Check sheet for the drawn part. Datum: minimum x, y, z corner. Units: mm. A direction names the side the tool comes from. Round coordinates to 2 decimals unless told otherwise and drop trailing zeros. Write each loop counter-clockwise with the first axis right and the second up, starting at its lowest first coordinate (ties: lowest second). Pieces come first, ordered by that corner, then holes. Notation, with made-up numbers: (6, 65) - (28, 65) arc R28 cw to (28, 95) - close; hole circle Ø10 at (-26, -33.75). An arc over 180 degrees is marked (long way). Answer as a JSON object with one key per item and string values.
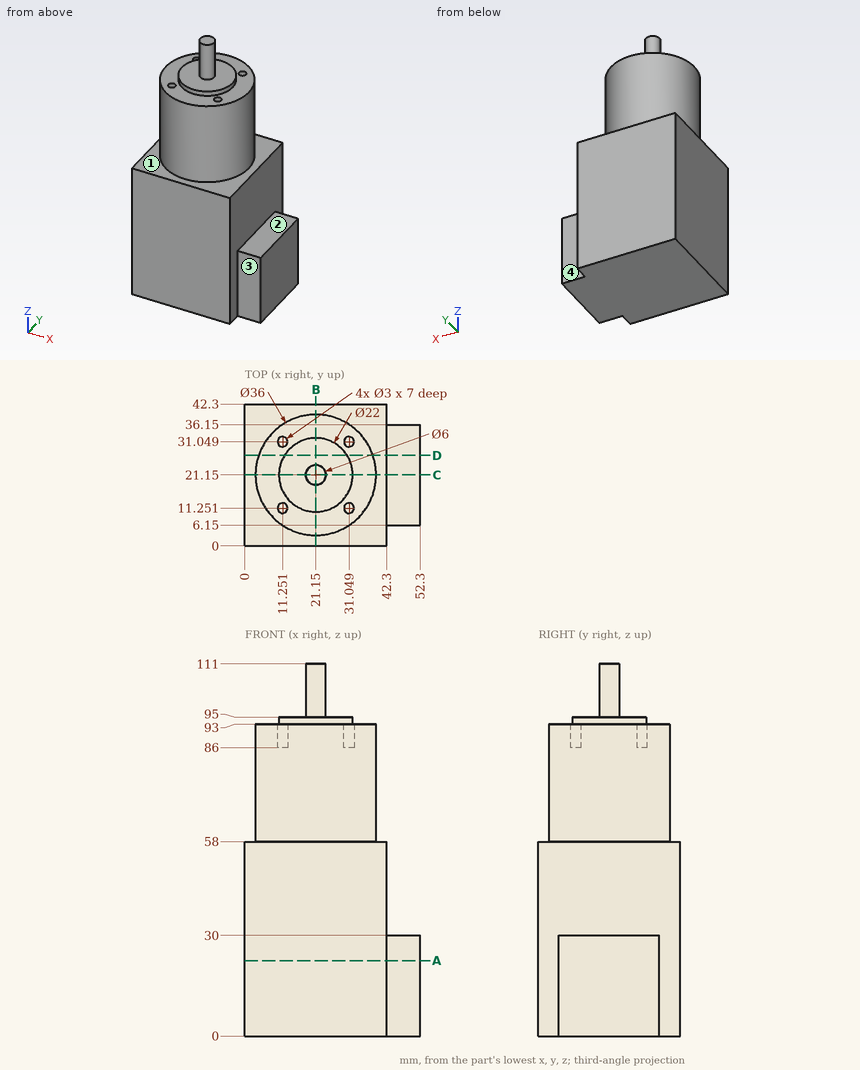
1. Cross-section at A-A (z = 22.5). Record the boundary of the cut face in (x, y), plus the area to 3 significant figures.
Completed:
{"outline": "(0, 0) - (42.3, 0) - (42.3, 6.15) - (52.3, 6.15) - (52.3, 36.15) - (42.3, 36.15) - (42.3, 42.3) - (0, 42.3) - close", "area": "2,090 mm^2"}
2. Material ranges on probe 1 along Z at (x, y) = (34, 6.5); probe 2 along Z at (x, y) = (26, 32); probe 3 along X at (y, z) = (5.5, 14.5), recorded low to high. Write a range as from..to.
Completed:
{"probe 1": "z = 0..58", "probe 2": "z = 0..93", "probe 3": "x = 0..42.3"}
3. Cross-section at B-B (x = 21.15). Record the boundary of the cut face in (y, z).
Completed:
{"outline": "(0, 0) - (42.3, 0) - (42.3, 58) - (39.15, 58) - (39.15, 93) - (32.15, 93) - (32.15, 95) - (24.15, 95) - (24.15, 111) - (18.15, 111) - (18.15, 95) - (10.15, 95) - (10.15, 93) - (3.15, 93) - (3.15, 58) - (0, 58) - close"}
4. Go/stop test with flat-tipped pins: pin 1 (5 mm diameter, centred on x = 48, z = 12.5, fed in from -Y); pin 2 (3.5 mm diameter, centred on x = 31.05, y = 11.25, fed in from +Z); pin 3 (1.5 mm diameter, centred on x = 31, y = 11.5, fed in from +Z). Record where each tip stops, or that it passes through.
Completed:
{"pin 1": "stops at y = 6.15", "pin 2": "stops at z = 93", "pin 3": "stops at z = 86"}
5. Access from +Z, -Z, +X, -X, +Y, -Y to the whole of each face (thin tool, end or side, straight path). Record for the marked faces 1, 2, 3 and 4.
Completed:
{"face 1": "+Z", "face 2": "+Z, +X, +Y, -Y", "face 3": "+Z, -Z, +X, -Y", "face 4": "+Z, -Z, +X, +Y"}
6. Cross-section at C-C (y = 21.15). Record the boundary of the cut face in (x, z).
Completed:
{"outline": "(0, 0) - (52.3, 0) - (52.3, 30) - (42.3, 30) - (42.3, 58) - (39.15, 58) - (39.15, 93) - (32.15, 93) - (32.15, 95) - (24.15, 95) - (24.15, 111) - (18.15, 111) - (18.15, 95) - (10.15, 95) - (10.15, 93) - (3.15, 93) - (3.15, 58) - (0, 58) - close"}
7. Cross-section at D-D (y = 27). Record the boundary of the cut face in (x, z) (1 decimal), plus the area to 3 significant figures.
Completed:
{"outline": "(0, 0) - (52.3, 0) - (52.3, 30) - (42.3, 30) - (42.3, 58) - (38.2, 58) - (38.2, 93) - (30.5, 93) - (30.5, 95) - (11.8, 95) - (11.8, 93) - (4.1, 93) - (4.1, 58) - (0, 58) - close", "area": "3,980 mm^2"}
